Geometry check sheet. Reference: the model listing, model coordinates, mm. Round coordinates to 2 decimals unless told otherwise and drop trailing zeros. One line per item, written item: value. Start each with the question number.
1. Release check for a two-part mould opening along X. For faces 1 (the flat face through (10, 138, -7)), 2 (the flat face through (2, 280, 2)), 3 (the flat face through (-10, 138, 7)), 4 (the cylindrical face through (-0.54, 138.04, 2.44)) record: pulls with the +X half, pulls with the -X half, needs draft (parallel to the pull), parting line crosses it, or undercut.
2. Scan lines: probe 1 along X at (y, z) = (253.5, -7.5); probe 2 along X at (y, z) = (182, 0). Record each from-to range of solid material in increasing order. Write a range as [from, to].
3. Depth check by flat-ended pin: P1, Ø3, axis at y = 169.5, z = -2.5, coming from the +X side; P2, Ø3, axis at y = 131, z = -4, coming from the +X side; P3, Ø1.5, axis at y = 74, z = -2.5, coming from the -X side; P4, Ø0.9, axis at x = 1.5, y = 158.5, coming from the -Z side. Enter the tip coordinate at first touch or a pass-through.
from build123d import *

# Parameters (mm, degrees)
ESQUISSE1_R      = 2.5
EXTRUSION1_DEPTH = 280
CONG_1_R         = 0.75


with BuildPart() as part:
    # Esquisse1 → Extrusion1 (new body)
    with BuildSketch(Plane(origin=(0, 0, 0), x_dir=(1, 0, 0), z_dir=(0, 1, 0))):
        Polygon((0, 4), (-0.5, 4.5), (-3.439339828, 4.5), (-6.439339828, 7.5), (-6.439339828, 8.5), (-3, 8.5), (-4.5, 10), (-10, 10), (-10, 4.5), (-8.5, 3), (-8.5, 6.439339828), (-7.5, 6.439339828), (-4.5, 3.439339828), (-4.5, 0.5), (-4, 0), (-4.5, -0.5), (-4.5, -3.439339828), (-7.5, -6.439339828), (-8.5, -6.439339828), (-8.5, -3), (-10, -4.5), (-10, -10), (-4.5, -10), (-3, -8.5), (-6.439339828, -8.5), (-6.439339828, -7.5), (-3.439339828, -4.5), (-0.5, -4.5), (0, -4), (0.5, -4.5), (3.439339828, -4.5), (6.439339828, -7.5), (6.439339828, -8.5), (3, -8.5), (4.5, -10), (10, -10), (10, -4.5), (8.5, -3), (8.5, -6.439339828), (7.5, -6.439339828), (4.5, -3.439339828), (4.5, -0.5), (4, 0), (4.5, 0.5), (4.5, 3.439339828), (7.5, 6.439339828), (8.5, 6.439339828), (8.5, 3), (10, 4.5), (10, 10), (4.5, 10), (3, 8.5), (6.439339828, 8.5), (6.439339828, 7.5), (3.439339828, 4.5), (0.5, 4.5), align=None)
        Circle(ESQUISSE1_R, mode=Mode.SUBTRACT)
    extrude(amount=EXTRUSION1_DEPTH)

    # Congé1
    cong_1_edges = [part.edges().sort_by_distance(p)[0] for p in [
        (6.439339828, 140, -8.5),
        (10, 140, -10),
        (8.5, 140, -6.439339828),
        (8.5, 140, 6.439339828),
        (10, 140, 10),
        (6.439339828, 140, 8.5),
        (-6.439339828, 140, 8.5),
        (-10, 140, 10),
        (-8.5, 140, 6.439339828),
        (-8.5, 140, -6.439339828),
        (-10, 140, -10),
        (-6.439339828, 140, -8.5),
    ]]
    fillet(cong_1_edges, radius=CONG_1_R)


solid = part.part
Result sheet:
1. face 1: pulls with the +X half
1. face 2: needs draft
1. face 3: pulls with the -X half
1. face 4: undercut
2. probe 1: x = [-10, -6.44], [6.44, 10]
2. probe 2: x = [-4, -2.5], [2.5, 4]
3. P1: stops at x = 9.5
3. P2: stops at x = 10
3. P3: stops at x = -8.75
3. P4: stops at z = -4.5
